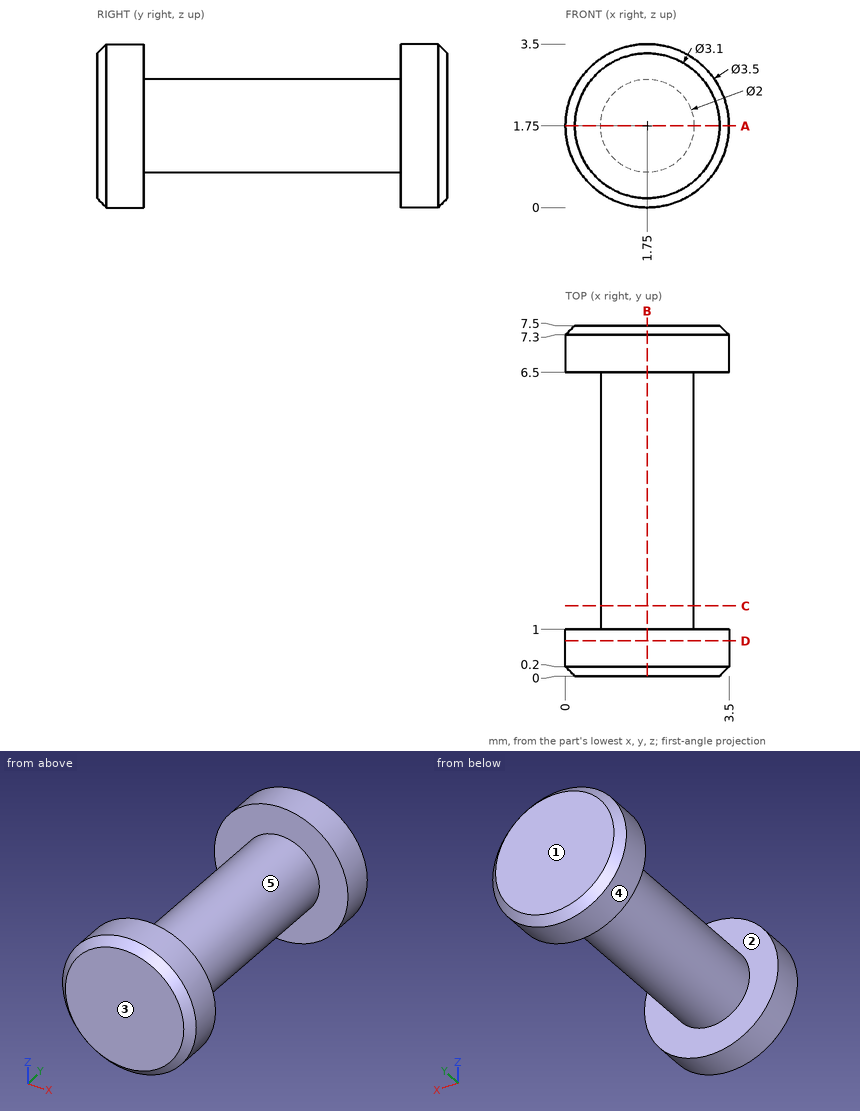
Geometry check sheet. Reference: drawing and pictorial views, mm from the part's lowest x, y, z. A direction names the side the tool comes from. Give positions to 0.01 mm unless a question says otherwise; leave off trailing zeros. Order: outer loops, then holes, each group sorted by start corner. A loop starts at its lowest first (then second) coordinate and runs counter-clockwise, first axis right, second up. Notation, with made-up numbers: M 6.5,-36.75 L 23.5,-36.75 A27 cw 23.5,-3.75 Z; hole C 11.5,19.25 d5. An arc over 180 degrees is marked long. Answer as a JSON object with one key per item and string values. Group by question number.
1) Access from +Z, -Z, +X, -X, +Y, -Y to the whole of each face (thin tool, end or side, straight path). Record for the marked faces 1 and 2.
2) Depth check by flat-ended pin: pin 1 Ø2 at (x, y) = (3, 6.5) entering from +Z; pin 2 Ø1.5 at (y, z) = (4, 1.5) entering from -X; pin 3 Ø1 at (x, y) = (2.5, 5) entering from -Z. Enter the tip coordinate at first touch or a pass-through.
3) Cross-section at A-A (z = 1.75). Enter the section's corners in (x, y), then the cut area to 3 significant figures.
4) Cross-section at C-C (y = 1.5). Enter the section's corners in (x, z), then the cut area to 3 significant figures.
5) Cross-section at B-B (x = 1.75). Enter the section's corners in (y, z), then the cut area to 3 significant figures.
6) Cross-section at D-D (y = 0.75). Enter the section's corners in (x, z), then the cut area to 3 significant figures.
7) Mould release check, pull along Y, two halves, no side actions. Record for the marked faces 3, 4 and 5: released by +Y, released by -Y, zero draft, split by the parting line, or undercut.
8) Scan lines: line 1 along Y through (x, z) = (0.65, 1.7); line 2 along X through (y, z) = (5, 1.8). Record each from-to range of solid material in increasing order. Write a range as [from, to].
Result sheet:
{
 "1": {"face 1": "+Z, -Z, +X, -X, +Y", "face 2": "none"},
 "2": {"pin 1": "stops at z = 3.48", "pin 2": "stops at x = 0.75", "pin 3": "stops at z = 0.78"},
 "3": {"outline": "M 0,0.2 L 0.2,0 L 3.3,0 L 3.5,0.2 L 3.5,1 L 2.75,1 L 2.75,6.5 L 3.5,6.5 L 3.5,7.3 L 3.3,7.5 L 0.2,7.5 L 0,7.3 L 0,6.5 L 0.75,6.5 L 0.75,1 L 0,1 Z", "area": "17.9 mm2"},
 "4": {"outline": "C 1.75,1.75 d2", "area": "3.14 mm2"},
 "5": {"outline": "M 0,0.2 L 0.2,0 L 1,0 L 1,0.75 L 6.5,0.75 L 6.5,0 L 7.3,0 L 7.5,0.2 L 7.5,3.3 L 7.3,3.5 L 6.5,3.5 L 6.5,2.75 L 1,2.75 L 1,3.5 L 0.2,3.5 L 0,3.3 Z", "area": "17.9 mm2"},
 "6": {"outline": "C 1.75,1.75 d3.5", "area": "9.62 mm2"},
 "7": {"face 3": "released by -Y", "face 4": "zero draft", "face 5": "undercut"},
 "8": {"line 1": "y = [0, 1], [6.5, 7.5]", "line 2": "x = [0.75, 2.75]"}
}
